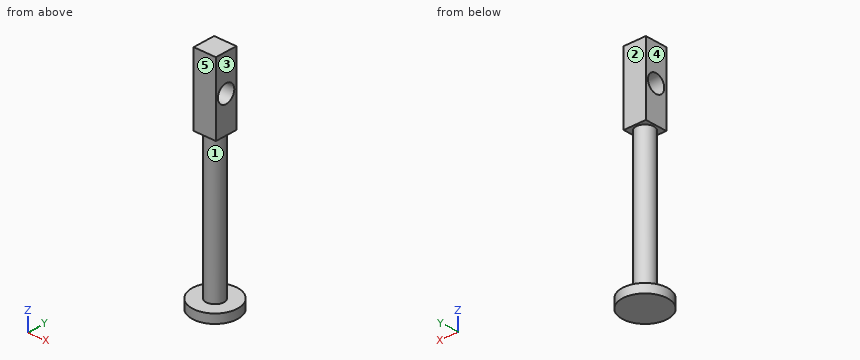
```python
from build123d import *

# Parameters (mm, degrees)
SKETCH1_R           = 12.7
BOSS_EXTRUDE1_DEPTH = 5
SKETCH2_R           = 5
BOSS_EXTRUDE3_DEPTH = 80
SKETCH3_W           = 12.446
SKETCH3_H           = 12.5
BOSS_EXTRUDE4_DEPTH = 40
SKETCH4_R           = 5
CUT_EXTRUDE1_DEPTH  = 128.060497122


with BuildPart() as part:
    # Sketch1 → Boss-Extrude1 (new body)
    with BuildSketch(Plane.XY):
        Circle(SKETCH1_R)
    extrude(amount=BOSS_EXTRUDE1_DEPTH)

    # Sketch2 → Boss-Extrude3 (add)
    with BuildSketch(Plane.XY.offset(5)):
        Circle(SKETCH2_R)
    extrude(amount=BOSS_EXTRUDE3_DEPTH)

    # Sketch3 → Boss-Extrude4 (add)
    with BuildSketch(Plane.XY.offset(85)):
        Rectangle(SKETCH3_W, SKETCH3_H)
    extrude(amount=BOSS_EXTRUDE4_DEPTH)

    # Sketch4 → Cut-Extrude1 (cut, through all)
    with BuildSketch(Plane.ZY.offset(6.223)):
        with Locations(Location((105, 0, 0), (0, 0, 270))):
            Circle(SKETCH4_R)
    extrude(amount=-CUT_EXTRUDE1_DEPTH, mode=Mode.SUBTRACT)


solid = part.part
```
Model file for the job. Use its own axes, mm. Face numbers are marked on the shaded views. A direction names the side the tool comes from. Give positions to 0.01 mm unless a question says otherwise; leave off trailing zeros. Write each loop counter-clockwise with the first axis right and the second up, starting at its lowest first coordinate (ties: lowest second). Pieces come first, ordered by that corner, then holes. Notation, with made-up numbers: (34.25, 35.25) -> (68.25, 35.25) arc R24 cw to (68.25, 48.25) -> close; hole circle Ø7 at (52.5, -33). An arc over 180 degrees is marked (long way). Use CSV: the item, a comma, the result in double quotes. Start each with the question number.
1) Pin check, flat tips, straight feed: P1, Ø6, axis at x = -2.5, z = 108.5, coming from the -Y side; P2, Ø6, axis at x = 2, z = 114.5, coming from the +Y side; P3, Ø12, axis at y = -5.5, z = 33.5, coming from the +X side. Stop position of each tip, or through.
2) Cut at C-C on y = 0. List the corners of the cut face in (x, z).
3) Drill centre lines: L1, parallel to Z at x = 1, y = 0; L2, parallel to Z at x = 4.75, y = -9.5; L3, parallel to X at y = 0, z = 116.5. Where is each one in solid material? Low to high.
4) Cut at D-D on z = 34. List the corners of the cut face in (x, y), plus the area to 3 significant figures.
5) Cut at A-A on z = 105. List the corners of the cut face in (x, y).
6) Tool access for the marked faces 1, 2, 3, 4 and 5: list every direction of +Z, -Z, +X, -X, +Y, -Y with a clear straight run to the whole face (end or side of a thin tool).
7) Cut at B-B on x = 0. List the corners of the cut face in (y, z).
Final values:
1,P1,"stops at y = -6.25"
1,P2,"stops at y = 6.25"
1,P3,"stops at x = 5"
2,outline,"(-12.7, 0) -> (12.7, 0) -> (12.7, 5) -> (5, 5) -> (5, 85) -> (6.22, 85) -> (6.22, 100) -> (-6.22, 100) -> (-6.22, 85) -> (-5, 85) -> (-5, 5) -> (-12.7, 5) -> close; (-6.22, 110) -> (6.22, 110) -> (6.22, 125) -> (-6.22, 125) -> close"
3,L1,"z = 0 to 100, 110 to 125"
3,L2,"z = 0 to 5"
3,L3,"x = -6.22 to 6.22"
4,outline,"circle Ø10 at (0, 0)"
4,area,"78.5 mm2"
5,outline,"(-6.22, -6.25) -> (6.22, -6.25) -> (6.22, -5) -> (-6.22, -5) -> close; (-6.22, 5) -> (6.22, 5) -> (6.22, 6.25) -> (-6.22, 6.25) -> close"
6,face 1,"none"
6,face 2,"+Z, +X, -X, +Y"
6,face 3,"+Z, +X, +Y, -Y"
6,face 4,"+Z, -X, +Y, -Y"
6,face 5,"+Z, +X, -X, -Y"
7,outline,"(-12.7, 0) -> (12.7, 0) -> (12.7, 5) -> (5, 5) -> (5, 85) -> (6.25, 85) -> (6.25, 125) -> (-6.25, 125) -> (-6.25, 85) -> (-5, 85) -> (-5, 5) -> (-12.7, 5) -> close; hole circle Ø10 at (0, 105)"
